Source: three-view drawing plus pictorial views. Frame: mm from the lowest corner of the part. A direction names the side the tool comes from. Coordinates: 2 decimals unless noted, no trailing zeros. Order: outer loops, then holes, each group sorted by start corner. A loop starts at its lowest first (then second) coordinate and runs counter-clockwise, first axis right, second up. Notation, with made-up numbers: M 52.25,83.5 L 104.25,83.5 A8 cw 104.25,98.5 Z; hole C 75.25,64.25 d3. An arc over 180 degrees is marked long. Write item = value, one per line. Start each with the question number.
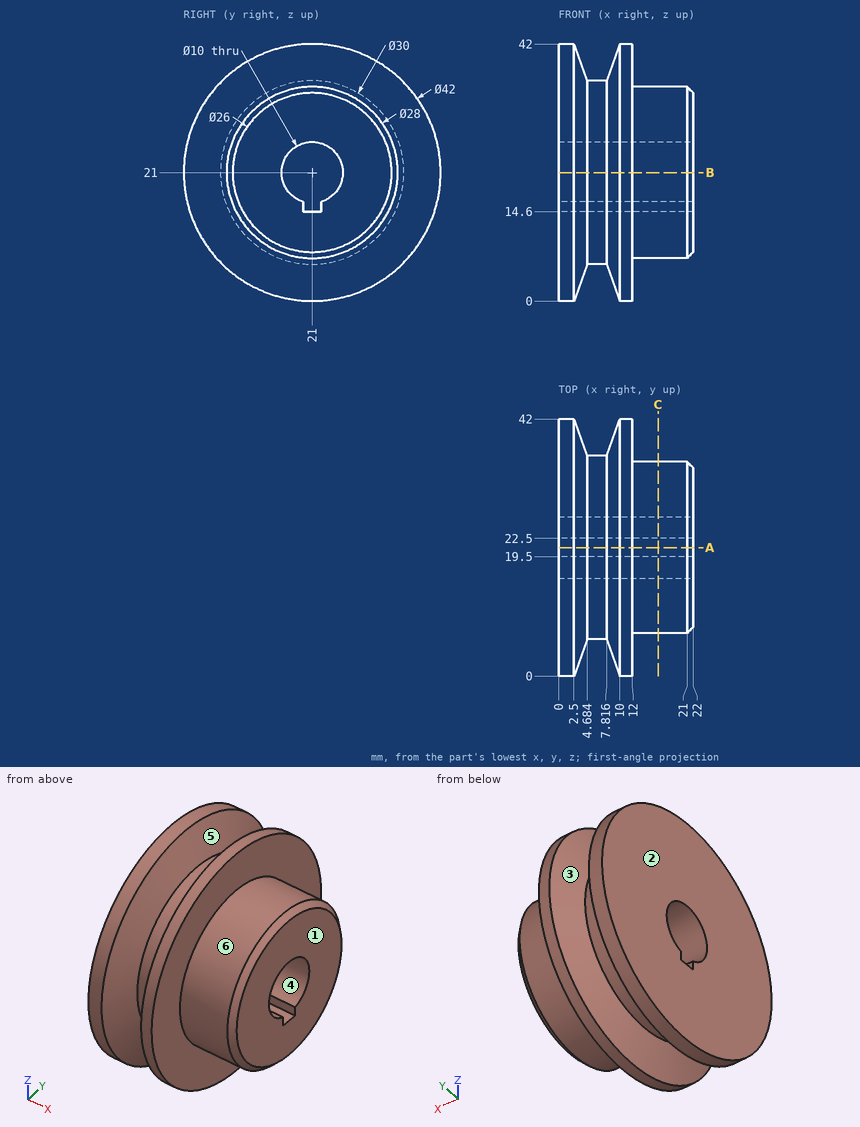
Item 1: Section query C-C on x = 16.25. Output: boundary loops of the cut face in (y, z).
Item 2: Section query B-B on z = 21. Output: boundary loops of the cut face in (x, y).
Item 3: First-contact query: pin 1 (5 mm diameter, centred on x = 8.5, y = 9, fed in from -Z); pin 2 (2 mm diameter, centred on y = 32.5, z = 37.5, fed in from +X); pin 3 (8 mm diameter, centred on x = 4.5, z = 7.5, fed in from -Y). Flat tips, straight axial feed; report the tip coordinate or a pass-through.
Item 4: Material intervals for probe 1 along Y at (x, z) = (11.25, 21); probe 2 along Z at (x, y) = (6, 21); probe 3 along Z at (x, y) = (12.5, 21), sorted ascending. Write a range as [from, to].
Item 5: Reachability of the marked faces 5 and 6 from +Z, -Z, +X, -X, +Y, -Y: full face, straight path, thin tool, end or side. Return the list, or none.
Item 6: Section query A-A on y = 21. Output: boundary loops of the cut face in (x, z).
Item 7: Draft query along X for the marked faces 1, 2, 3 and 4. Return one class per face: pulls with the +X half, pulls with the -X half, needs draft (parallel to the pull), parting line crosses it, or undercut.
Ans:
q1.outline = C 21,21 d28; hole M 19.5,14.6 L 22.5,14.6 L 22.5,16.23 A5 ccw long 19.5,16.23 Z
q2.outline = M 0,0 L 2.5,0 L 4.68,6 L 7.82,6 L 10,0 L 12,0 L 12,7 L 21,7 L 22,8 L 22,16 L 0,16 Z; M 0,26 L 22,26 L 22,34 L 21,35 L 12,35 L 12,42 L 10,42 L 7.82,36 L 4.68,36 L 2.5,42 L 0,42 Z
q3.pin_1 = 2.53
q3.pin_2 = 12
q3.pin_3 = 2.55
q4.probe_1 = [0, 16], [26, 42]
q4.probe_2 = [6, 14.6], [26, 36]
q4.probe_3 = [7, 14.6], [26, 35]
q5.face_5 = none
q5.face_6 = +X
q6.outline = M 0,0 L 2.5,0 L 4.68,6 L 7.82,6 L 10,0 L 12,0 L 12,7 L 21,7 L 22,8 L 22,14.6 L 0,14.6 Z; M 0,26 L 22,26 L 22,34 L 21,35 L 12,35 L 12,42 L 10,42 L 7.82,36 L 4.68,36 L 2.5,42 L 0,42 Z
q7.face_1 = pulls with the +X half
q7.face_2 = pulls with the -X half
q7.face_3 = undercut
q7.face_4 = needs draft
